CAD build for the part. Positions are in the model's coordinates, mm. A direction names the side the tool comes from. Coordinates: 2 decimals unless noted, no trailing zeros. Loops run counter-clockwise (first coordinate to the right, second up) from the corner with the lowest first, then second, coordinate; pieces in that order, holes last. Notation, with made-up numbers: (63, 71.25) -> (99, 71.25) arc R26 ccw to (99, 95.25) -> close; hole circle Ø6 at (55, 65.5). An arc over 180 degrees is marked (long way). Write item = value, one per line. Start each with the question number.
(1) Drill centre lines: line 1 (Z direction, x = 665.84, y = 15); line 2 (Z direction, x = -335.5, y = 28.5); line 3 (X direction, y = 45, z = -9). Where is each one in solid material? Low to high. Write a range as from..to.
(2) Tool access for faces 1 (the face through (-581, 54, 119)), 2 (the face through (-481, -30, -199)), 3 (the face through (674, -30, 150)): list every direction of +Z, -Z, +X, -X, +Y, -Y with a clear straight run to the whole face (end or side of a thin tool).
(3) Band-saw the part on A-A (x = 350). Write the cut outline in (y, z).
(4) Pull direction X, two halves, no side cores. Call faces 4 (the face through (-2, 48, -80)), 5 (the face through (750, 14, 3)), 6 (the face through (-557, -30, 150)): +X half, -X half, draft (parallel to the pull), parting line (faces both ways), or undercut.
(5) Band-saw the part on B-B (y = -35). Write the cut outline in (x, z), and give its area (3 significant figures).
(6) Band-saw the part on C-C (z = 214.5). Write the cut outline in (x, y), and give its area (3 significant figures).
(7) Flat gauge pins, fed straight in: P1, Ø4.5, axis at x = 253.75, z = 82.5, coming from the +Y side; P2, Ø3, axis at x = 308, z = 47, coming from the +Y side; P3, Ø6, axis at x = 297.5, z = -52.5, coming from the -Y side. Where does each tip first touch, or does it go through?
(8) Band-saw the part on D-D (x = -457). Write the cut outline in (y, z).
```python
from build123d import *

# Parameters (mm, degrees)
SKETCH19_W               = 1030
SKETCH19_H               = 180
SKETCH19_W_2             = 1000
SKETCH19_H_2             = 150
BOSS_EXTRUDE2_DEPTH      = 48
SKETCH22_W               = 1030
SKETCH22_H               = 180
BOSS_EXTRUDE3_DEPTH      = 10
BOSS_EXTRUDE4_DEPTH      = 56
BOSS_EXTRUDE4_DEPTH_BACK = 10
SKETCH23_W               = 1500
SKETCH23_H               = 500
SKETCH23_W_2             = 1030
SKETCH23_H_2             = 180
CUT_EXTRUDE6_START       = 48
SKETCH26_R               = 1.65
CUT_EXTRUDE6_DEPTH       = 20
LPATTERN1_COUNT          = 5
LPATTERN1_PITCH          = 253.75
SKETCH28_R               = 2.3
SKETCH28_R_2             = 57.7
CUT_EXTRUDE7_DEPTH       = 793.55031386
LPATTERN2_COUNT          = 2
LPATTERN2_PITCH          = 350
LPATTERN2_COL_COUNT      = 2
LPATTERN2_COL_PITCH      = 350
CUT_EXTRUDE8_START       = 48
SKETCH27_R               = 1.65
CUT_EXTRUDE8_DEPTH       = 20
CUT_EXTRUDE9_START       = -56
CUT_EXTRUDE9_DEPTH       = 2
CUT_EXTRUDE10_START      = 56
CUT_EXTRUDE10_DEPTH      = 2
CUT_EXTRUDE11_DEPTH      = 793.55031386
CUT_EXTRUDE11_DEPTH_BACK = 793.55031386
SKETCH33_R               = 2.35
CUT_EXTRUDE12_DEPTH      = 793.55031386
CUT_EXTRUDE12_DEPTH_BACK = 793.55031386
SKETCH34_W               = 190.830831748
SKETCH34_H               = 540.530008981
SKETCH29_W               = 150
SKETCH29_H               = 100
BOSS_EXTRUDE5_DEPTH      = 50


with BuildPart() as part:
    # Sketch19 → Boss-Extrude2 (new body)
    with BuildSketch(Plane(origin=(0, 0, 0), x_dir=(1, 0, 0), z_dir=(0, 1, 0))):
        Rectangle(SKETCH19_W, SKETCH19_H)
        Rectangle(SKETCH19_W_2, SKETCH19_H_2, mode=Mode.SUBTRACT)
    extrude(amount=BOSS_EXTRUDE2_DEPTH)

    # Sketch22 → Boss-Extrude3 (add)
    with BuildSketch(Plane(origin=(0, 0, 0), x_dir=(1, 0, 0), z_dir=(0, 1, 0))):
        Rectangle(SKETCH22_W, SKETCH22_H)
    extrude(amount=-BOSS_EXTRUDE3_DEPTH)

    # Sketch23 → Boss-Extrude4 (add, two sides: drawn at the far end of the back side and taken through both)
    with BuildSketch(Plane(origin=(0, 0, 0), x_dir=(1, 0, 0), z_dir=(0, 1, 0)).offset(-BOSS_EXTRUDE4_DEPTH_BACK)):
        Rectangle(SKETCH23_W, SKETCH23_H)
        Rectangle(SKETCH23_W_2, SKETCH23_H_2, mode=Mode.SUBTRACT)
    extrude(amount=BOSS_EXTRUDE4_DEPTH + BOSS_EXTRUDE4_DEPTH_BACK)

    # Sketch26 → Cut-Extrude6 (cut)
    with BuildSketch(Plane(origin=(0, 0, 0), x_dir=(1, 0, 0), z_dir=(0, 1, 0)).offset(CUT_EXTRUDE6_START)):
        with Locations(Location((-507.5, -82.5, 0), (0, 0, 90))):
            Circle(SKETCH26_R)
        with Locations(Location((-507.5, 82.5, 0), (0, 0, 90))):
            Circle(SKETCH26_R)
    cut_extrude6 = extrude(amount=-CUT_EXTRUDE6_DEPTH, mode=Mode.SUBTRACT)

    # LPattern1: Cut-Extrude6 ×5
    with Locations(*[(i * LPATTERN1_PITCH, 0, 0) for i in range(1, LPATTERN1_COUNT)]):
        add(cut_extrude6, mode=Mode.SUBTRACT)

    # Sketch28 → Cut-Extrude7 (cut, symmetric)
    with BuildSketch(Plane(origin=(0, 0, 0), x_dir=(1, 0, 0), z_dir=(0, 1, 0))):
        with Locations(Location((-52.5, 52.5, 0), (0, 0, 270))):
            Circle(SKETCH28_R)
        with Locations(Location((52.5, 52.5, 0), (0, 0, 270))):
            Circle(SKETCH28_R)
        with Locations(Location((52.5, -52.5, 0), (0, 0, 270))):
            Circle(SKETCH28_R)
        with Locations(Location((-52.5, -52.5, 0), (0, 0, 270))):
            Circle(SKETCH28_R)
        with Locations(Location((0, 0, 0), (0, 0, 270))):
            Circle(SKETCH28_R_2)
    cut_extrude7 = extrude(amount=CUT_EXTRUDE7_DEPTH, both=True, mode=Mode.SUBTRACT)

    # LPattern2: Cut-Extrude7 ×2
    with Locations(*[(-i * LPATTERN2_PITCH, 0, 0) for i in range(1, LPATTERN2_COUNT)]):
        add(cut_extrude7, mode=Mode.SUBTRACT)

    # LPattern2 col: Cut-Extrude7 ×2
    with Locations(*[(i * LPATTERN2_COL_PITCH, 0, 0) for i in range(1, LPATTERN2_COL_COUNT)]):
        add(cut_extrude7, mode=Mode.SUBTRACT)

    # Sketch27 → Cut-Extrude8 (cut)
    with BuildSketch(Plane(origin=(0, 0, 0), x_dir=(1, 0, 0), z_dir=(0, 1, 0)).offset(CUT_EXTRUDE8_START)):
        with Locations(Location((507.5, 0, 0), (0, 0, 90))):
            Circle(SKETCH27_R)
        with Locations(Location((-507.5, 47.503341606, 0), (0, 0, 90))):
            Circle(SKETCH27_R)
        with Locations(Location((-507.5, -42.394481769, 0), (0, 0, 90))):
            Circle(SKETCH27_R)
    extrude(amount=-CUT_EXTRUDE8_DEPTH, mode=Mode.SUBTRACT)

    # Sketch30 → Cut-Extrude9 (cut)
    with BuildSketch(Plane.XZ.offset(CUT_EXTRUDE9_START)):
        with BuildLine():
            Line((571.5, -147.92), (714.5, -147.92))
            ThreePointArc((714.5, -147.92), (715.207106781, -147.627106781), (715.5, -146.92))
            Line((715.5, -146.92), (715.5, -89.92))
            ThreePointArc((715.5, -89.92), (715.207106781, -89.212893219), (714.5, -88.92))
            Line((714.5, -88.92), (571.5, -88.92))
            ThreePointArc((571.5, -88.92), (567.964466094, -90.384466094), (566.5, -93.92))
            Line((566.5, -93.92), (566.5, -142.92))
            ThreePointArc((566.5, -142.92), (567.964466094, -146.455533906), (571.5, -147.92))
        make_face()
    cut_extrude9 = extrude(amount=CUT_EXTRUDE9_DEPTH, mode=Mode.SUBTRACT)

    # Mirror1: Cut-Extrude9 across plane
    add(cut_extrude9.mirror(Plane.XY), mode=Mode.SUBTRACT)

    # Sketch32 → Cut-Extrude10 (cut)
    with BuildSketch(Plane(origin=(0, 0, 0), x_dir=(1, 0, 0), z_dir=(0, 1, 0)).offset(CUT_EXTRUDE10_START)):
        with BuildLine():
            Line((-591.5, 147.92), (-571.5, 147.92))
            ThreePointArc((-571.5, 147.92), (-567.964466094, 146.455533906), (-566.5, 142.92))
            Line((-566.5, 142.92), (-566.5, 93.92))
            ThreePointArc((-566.5, 93.92), (-567.964466094, 90.384466094), (-571.5, 88.92))
            Line((-571.5, 88.92), (-591.5, 88.92))
            ThreePointArc((-591.5, 88.92), (-595.035533906, 90.384466094), (-596.5, 93.92))
            Line((-596.5, 93.92), (-596.5, 142.92))
            ThreePointArc((-596.5, 142.92), (-595.035533906, 146.455533906), (-591.5, 147.92))
        make_face()
    cut_extrude10 = extrude(amount=-CUT_EXTRUDE10_DEPTH, mode=Mode.SUBTRACT)

    # Mirror2: Cut-Extrude10 across plane
    add(cut_extrude10.mirror(Plane.XY), mode=Mode.SUBTRACT)

    # Sketch33 → Cut-Extrude11 (cut, two sides: drawn at the far end of the back side and taken through both)
    with BuildSketch(Plane(origin=(0, 0, 0), x_dir=(1, 0, 0), z_dir=(0, 1, 0)).offset(-CUT_EXTRUDE11_DEPTH_BACK)):
        with Locations(Location((-581.5, 108.58, 0), (0, 0, 270))):
            Circle(SKETCH33_R)
        with Locations(Location((-581.5, -108.59, 0), (0, 0, 270))):
            Circle(SKETCH33_R)
        with Locations(Location((-581.5, 128.25, 0), (0, 0, 270))):
            Circle(SKETCH33_R)
        with Locations(Location((-581.5, -128.26, 0), (0, 0, 270))):
            Circle(SKETCH33_R)
        with Locations(Location((616.17, -118.42, 0), (0, 0, 270))):
            Circle(SKETCH33_R)
        with Locations(Location((665.84, -118.42, 0), (0, 0, 270))):
            Circle(SKETCH33_R)
        with Locations(Location((616.17, 118.42, 0), (0, 0, 270))):
            Circle(SKETCH33_R)
        with Locations(Location((665.84, 118.42, 0), (0, 0, 270))):
            Circle(SKETCH33_R)
    extrude(amount=CUT_EXTRUDE11_DEPTH + CUT_EXTRUDE11_DEPTH_BACK, mode=Mode.SUBTRACT)

    # Sketch34 → Cut-Extrude12 (cut, two sides: drawn at the far end of the back side and taken through both)
    with BuildSketch(Plane(origin=(0, 0, 0), x_dir=(1, 0, 0), z_dir=(0, 1, 0)).offset(-CUT_EXTRUDE12_DEPTH_BACK)):
        with Locations((-726.415415874, 20.265004491)):
            Rectangle(SKETCH34_W, SKETCH34_H)
    extrude(amount=CUT_EXTRUDE12_DEPTH + CUT_EXTRUDE12_DEPTH_BACK, mode=Mode.SUBTRACT)

    # Sketch29 → Boss-Extrude5 (add)
    with BuildSketch(Plane(origin=(0, 0, 0), x_dir=(1, 0, 0), z_dir=(0, 1, 0))):
        with Locations((-556, -200)):
            Rectangle(SKETCH29_W, SKETCH29_H)
        with Locations((-556, 200)):
            Rectangle(SKETCH29_W, SKETCH29_H)
        with Locations((675, -200)):
            Rectangle(SKETCH29_W, SKETCH29_H)
        with Locations((675, 200)):
            Rectangle(SKETCH29_W, SKETCH29_H)
    extrude(amount=-BOSS_EXTRUDE5_DEPTH)


solid = part.part
```
Findings below:
q1.line_1 = -250..-120.77, -116.07..116.07, 120.77..250
q1.line_2 = -250..-75, 75..250
q1.line_3 = -631..-500, 500..750
q2.face_1 = +Y
q2.face_2 = +Z, -Z, -Y
q2.face_3 = +X, -X, -Y
q3.outline = (-10, -250) -> (56, -250) -> (56, -90) -> (48, -90) -> (48, -75) -> (0, -75) -> (0, -57.7) -> (-10, -57.7) -> close; (-10, 57.7) -> (0, 57.7) -> (0, 75) -> (48, 75) -> (48, 90) -> (56, 90) -> (56, 250) -> (-10, 250) -> close
q4.face_4 = undercut
q4.face_5 = +X half
q4.face_6 = draft
q5.outline = (-631, -250) -> (-481, -250) -> (-481, -150) -> (-631, -150) -> close; (-631, 150) -> (-481, 150) -> (-481, 250) -> (-631, 250) -> close; (600, -250) -> (750, -250) -> (750, -150) -> (600, -150) -> close; (600, 150) -> (750, 150) -> (750, 250) -> (600, 250) -> close
q5.area = 60,000 mm²
q6.outline = (-631, -50) -> (-481, -50) -> (-481, -10) -> (600, -10) -> (600, -50) -> (750, -50) -> (750, 56) -> (-631, 56) -> close
q6.area = 103,000 mm²
q7.P1 = 48
q7.P2 = 0
q7.P3 = -10
q8.outline = (-10, -250) -> (56, -250) -> (56, -90) -> (48, -90) -> (48, -75) -> (0, -75) -> (0, 75) -> (48, 75) -> (48, 90) -> (56, 90) -> (56, 250) -> (-10, 250) -> close
